Solid Edge part; units mm, degrees
sketch "Sketch1" plane through (0, 54.6395, 8.8452) normal (1, 0, 0) x (0, 1, 0)
  line L0 (-54, 10) -> (-37.3222, 10)
  arc A0 (-37.3222, 10) -> (-31.9318, 8.8298) centre (-37.3222, -3) cw
  line L1 (-24.4906, 5.4391) -> (-31.9318, 8.8298)
  arc A1 (-24.4906, 5.4391) -> (-22.1504, 1.8947) centre (-26.1492, 1.7992) cw
  line L2 (-22.1504, 1.8947) -> (-22.0635, -1.7414)
  arc A2 (-24.427, -5.4873) -> (-22.0635, -1.7414) centre (-26.0624, -1.8369) ccw
  line L3 (-31.9639, -8.8638) -> (-24.427, -5.4873)
  arc A3 (-37.2789, -10) -> (-31.9639, -8.8638) centre (-37.2789, 3) ccw
  line L4 (-54, -10) -> (-37.2789, -10)
  arc A4 (-54, -10) -> (-57, -7) centre (-54, -7) cw
  line L5 (-57, 7) -> (-57, -7)
  arc A5 (-54, 10) -> (-57, 7) centre (-54, 7) ccw
extrude "Protrusion1" add sketch "Sketch1" along normal mid plane 9
sketch "Sketch2" plane through (-45.6395, -10, -1.1548) normal (0, 0, -1) x (0, 1, 0)
  arc A0 (25.4838, 50.1395) -> (12.3551, 50.1395) centre (18.9194, 49.1395) cw
  line L0 (12.3551, 50.1395) -> (25.4838, 50.1395)
extrude "Cutout1" cut sketch "Sketch2" against normal up to next and the other way through all
hole "Hole_1" at (4.5, 26.8926, 8.9219) direction (-1, 0, 0) diameter 6 end up to next
sketch "Sketch3" plane through (-4.5, 15.1083, 8.8452) normal (-1, 0, 0) x (0, 1, 0)
  line L0 (-3.7608, 6) -> (-11.4688, 6)
  arc A0 (-11.4688, 6) -> (-13.4688, 4) centre (-11.4688, 4) ccw
  line L1 (-13.4688, 4) -> (-13.4688, -4)
  arc A1 (-13.4688, -4) -> (-11.4688, -6) centre (-11.4688, -4) ccw
  line L2 (-11.4688, -6) -> (-3.7781, -6)
  arc A2 (-3.7781, -6) -> (-1.7781, -4.0043) centre (-3.7781, -4) ccw
  line L3 (-1.7781, -4.0043) -> (-1.7608, 3.9957)
  arc A3 (-3.7608, 6) -> (-1.7608, 3.9957) centre (-3.7608, 4) cw
extrude "ExtrudedCutout_3" cut sketch "Sketch3" against normal blind 1 and the other way blind 11.7703
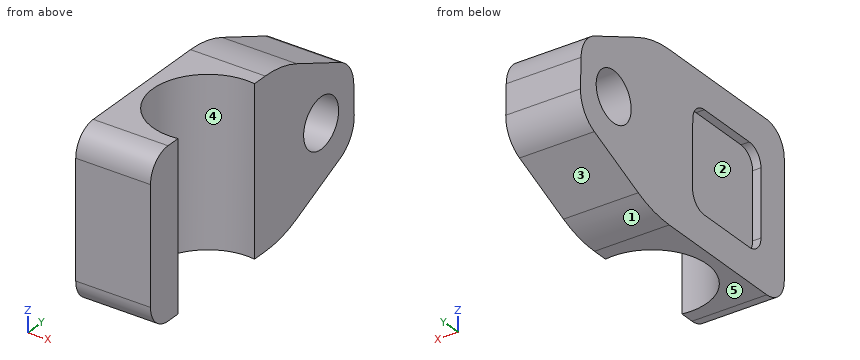
Can you work these out from the model? Positions are in its coordinate system, mm. Face numbers are marked on the shaded views. A direction names the side the tool comes from. Coordinates: 2 decimals unless noted, no trailing zeros. Write each loop counter-clockwise with the first axis right and the second up, starting at its lowest first coordinate (ties: lowest second). Pieces come first, ordered by that corner, then holes. Notation, with made-up numbers: (9.25, 45) - (35.25, 45) arc R30 cw to (35.25, 67) - close; hole circle Ø3 at (3.25, 40.5). An arc over 180 degrees is marked (long way). Return JSON: item names as keys, results as strings. Group by question number.
Item 1: If we section it at D-D (x = 2.75): Write out the boundary of the cut face in (y, z).
Item 2: Which directions (+Z, -Z, +X, -X, +Y, -Y) give clear straight access to the entire face, cutting with the end or side of a thin tool? Please do the marked faces 1 and 2.
Item 3: We'd pull the mould along Y, two halves only. Please class the marked faces 3, 4 and 5: pulls with the +Y half, pulls with the -Y half, needs draft (parallel to the pull), parting line crosses it, or undercut.
Item 4: I'm going to push flat-ended pins straight in: pin 1 Ø0.8 at (x, z) = (-4, 10.5) entering from +Y; pin 2 Ø5.5 at (y, z) = (26.89, 8.92) entering from +X. Where does each tip first touch, or does it pass through?
Item 5: Please list where these lines run through material, in increasing order: probe 1 along Y at (x, z) = (0, 8); probe 2 along Y at (x, z) = (1, 7.25); probe 3 along Y at (x, z) = (-2.25, 1.25).
Item 6: If we section it at C-C (z = 7.75): Write out the boundary of the cut face in (x, y), then the cut area to 3 significant figures.
Item 7: If we section it at A-A (x = 0.75): Write out the boundary of the cut face in (y, z).
Item 8: If we section it at B-B (y = 25.5): Write out the boundary of the cut face in (x, z), then the cut area to 3 significant figures.
Return value:
{
 "1": {"outline": "(-2.36, 1.85) arc R3 ccw to (0.64, -1.15) - (2.32, -1.15) - (2.32, 18.85) - (0.64, 18.85) arc R3 ccw to (-2.36, 15.85) - close; (15.52, -1.15) - (17.36, -1.15) arc R13 ccw to (22.68, -0.02) - (30.21, 3.36) arc R4 ccw to (32.58, 7.1) - (32.49, 10.74) arc R4 ccw to (30.15, 14.28) - (22.71, 17.67) arc R13 ccw to (17.32, 18.85) - (15.52, 18.85) - close; hole circle Ø6 at (26.89, 8.92)"},
 "2": {"face 1": "-Z, +X, -X, +Y", "face 2": "-X"},
 "3": {"face 3": "pulls with the +Y half", "face 4": "undercut", "face 5": "needs draft"},
 "4": {"pin 1": "stops at y = 32.5", "pin 2": "passes through"},
 "5": {"probe 1": "y = -2.36 to 3.28, 14.56 to 24.04, 29.75 to 32.55", "probe 2": "y = -2.36 to 2.77, 15.07 to 24.4, 29.38 to 32.57", "probe 3": "y = -2.3 to 5.6, 12.24 to 25.51"},
 "6": {"outline": "(-4.5, -2.36) - (4.5, -2.36) - (4.5, 2.36) arc R6.64 cw (long way) to (4.5, 15.48) - (4.5, 24.13) - (-4.5, 24.13) - (-4.5, 13.34) - (-3.5, 13.34) - (-3.5, 1.64) - (-4.5, 1.64) - close; (-4.5, 29.65) - (4.5, 29.65) - (4.5, 32.56) - (-4.5, 32.56) - close", "area": "170 mm^2"},
 "7": {"outline": "(-2.36, 1.85) arc R3 ccw to (0.64, -1.15) - (2.88, -1.15) - (2.88, 18.85) - (0.64, 18.85) arc R3 ccw to (-2.36, 15.85) - close; (14.96, -1.15) - (17.36, -1.15) arc R13 ccw to (22.68, -0.02) - (30.21, 3.36) arc R4 ccw to (32.58, 7.1) - (32.49, 10.74) arc R4 ccw to (30.15, 14.28) - (22.71, 17.67) arc R13 ccw to (17.32, 18.85) - (14.96, 18.85) - close; hole circle Ø6 at (26.89, 8.92)"},
 "8": {"outline": "(-4.5, 1.25) - (4.5, 1.25) - (4.5, 6.26) - (-4.5, 6.26) - close; (-4.5, 11.58) - (4.5, 11.58) - (4.5, 16.4) - (-4.5, 16.4) - close", "area": "88.6 mm^2"}
}
